Geometry: see drawing. Coordinates: mm, zero at the bounding-box minimum. A direction names the side the tool comes from. Give positions to 0.01 mm unless a question says otherwise; leave off trailing zeros. Loops run counter-clockwise (first coordinate to the right, second up) from the corner with the lowest first, then second, coordinate; pieces in that order, holes last. Notation, with made-up numbers: (71.25, 46) -> (79.25, 46) arc R36 cw to (79.25, 83) -> close; hole circle Ø2 at (3, 41.25). An arc over 180 degrees is marked (long way). Return JSON: item names as keys, results as strings. Group by question number.
(1) Cut plane B-B on z = 11. Return loops of the section in (x, y).
(2) Ray query, line 1 (X direction, y = 36.5, z = 9.5); line 2 (Y direction, x = 40, z = 22); line 3 (X direction, y = 13, z = 17.75). Return the intervals inside material, ascending. Write a range as from..to.
(3) Pin query (flat end, axial travel): pin 1 (5 mm diameter, centred on x = 8.5, z = 14.5, fed in from -Y); pin 2 (1 mm diameter, centred on y = 17.5, z = 3.5, fed in from -X). Return the tip coordinate at first contact, or that it passes through.
(4) Access query for the marked faces 1, 2 and 3. Directions: +Z, -Z, +X, -X, +Y, -Y. A direction counts if a zero-diameter tool reaches every point of the face in a straight line with its end or side. Return the directions, or none.
(5) Cut plane C-C on y = 35.5. Return loops of the section in (x, z), then the cut area to 3 significant figures.
(6) Cut plane A-A on x = 33.5. Return loops of the section in (y, z), then the cut area to 3 significant figures.
(7) Draft query along Y for the marked faces 4, 5 and 6. Return one class per face: released by +Y, released by -Y, zero draft, split by the parting line, or undercut.
(8) Cut plane D-D on y = 20. Return loops of the section in (x, z).
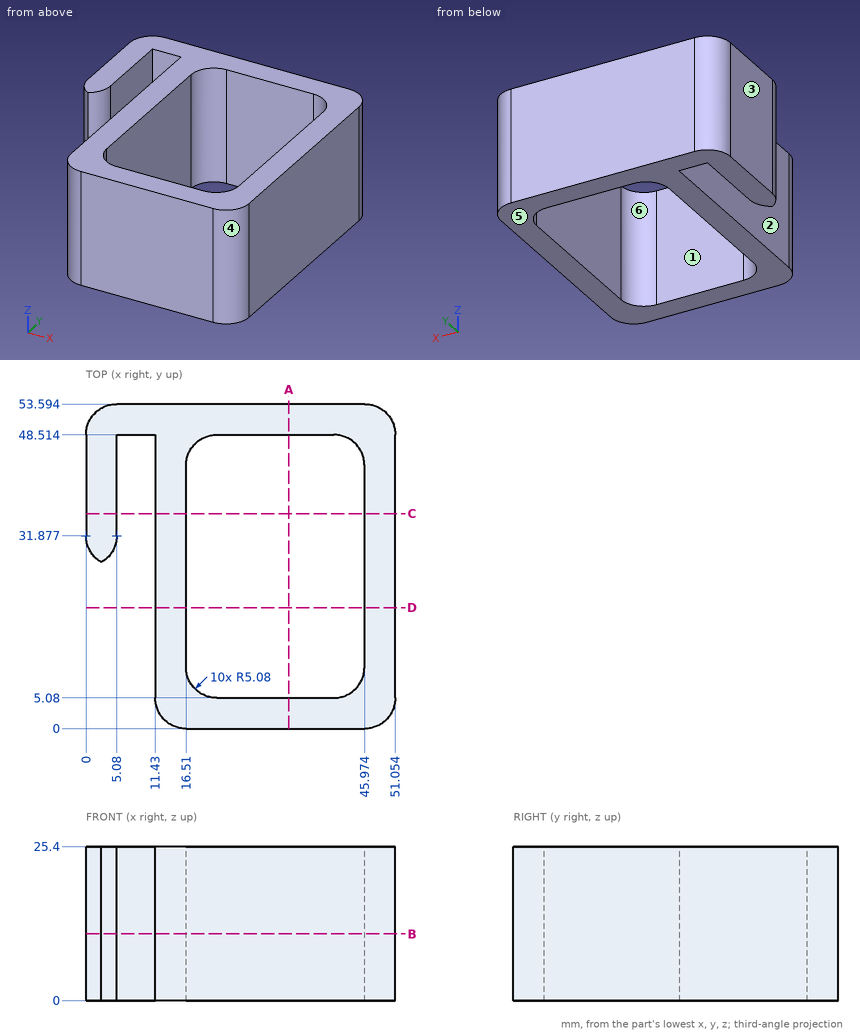
Answers:
{
 "1": {"outline": "(0, 31.88) arc R5.08 ccw to (2.54, 27.48) arc R5.08 ccw to (5.08, 31.88) -> (5.08, 48.51) -> (11.43, 48.51) -> (11.43, 5.08) arc R5.08 ccw to (16.51, 0) -> (45.97, 0) arc R5.08 ccw to (51.05, 5.08) -> (51.05, 48.51) arc R5.08 ccw to (45.97, 53.59) -> (5.08, 53.59) arc R5.08 ccw to (0, 48.51) -> close; hole (16.51, 10.16) arc R5.08 ccw to (21.59, 5.08) -> (40.89, 5.08) arc R5.08 ccw to (45.97, 10.16) -> (45.97, 43.43) arc R5.08 ccw to (40.89, 48.51) -> (21.59, 48.51) arc R5.08 ccw to (16.51, 43.43) -> close"},
 "2": {"line 1": "0..5.08, 11.43..16.51, 45.97..51.05", "line 2": "0..5.08, 48.51..53.59", "line 3": "11.43..16.51, 45.97..51.05"},
 "3": {"pin 1": "y = 48.51", "pin 2": "x = 11.43"},
 "4": {"face 1": "+Z, -Z", "face 2": "+Z, -Z, -Y", "face 3": "+Z, -Z, -X, +Y, -Y"},
 "5": {"outline": "(0, 0) -> (5.08, 0) -> (5.08, 25.4) -> (0, 25.4) -> close; (11.43, 0) -> (16.51, 0) -> (16.51, 25.4) -> (11.43, 25.4) -> close; (45.97, 0) -> (51.05, 0) -> (51.05, 25.4) -> (45.97, 25.4) -> close", "area": "387 mm²"},
 "6": {"outline": "(0, 0) -> (5.08, 0) -> (5.08, 25.4) -> (0, 25.4) -> close; (48.51, 0) -> (53.59, 0) -> (53.59, 25.4) -> (48.51, 25.4) -> close", "area": "258 mm²"},
 "7": {"face 4": "released by -Y", "face 5": "zero draft", "face 6": "undercut"},
 "8": {"outline": "(11.43, 0) -> (16.51, 0) -> (16.51, 25.4) -> (11.43, 25.4) -> close; (45.97, 0) -> (51.05, 0) -> (51.05, 25.4) -> (45.97, 25.4) -> close"}
}
